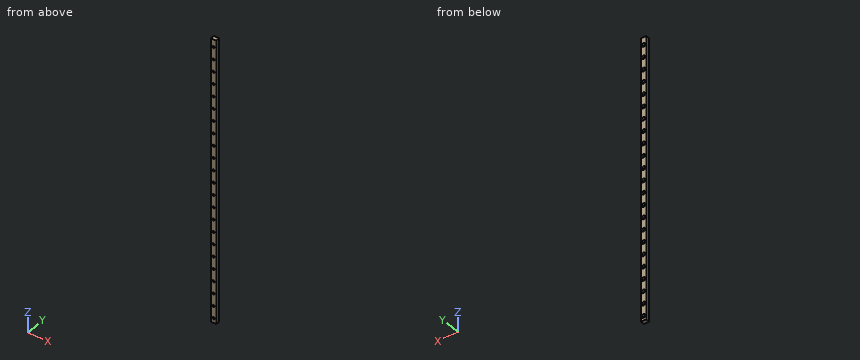
```python
from build123d import *

# Parameters (mm, degrees)
SKETCH_1_W          = 9
SKETCH_1_H          = 6.5
EXTRUDE_1_DEPTH     = 460
SKETCH_2_R          = 1.750000006
CUT_EXTRUDE_1_DEPTH = 371.819449874
SKETCH_3_R          = 3.000000006
CUT_EXTRUDE_2_DEPTH = 3.5


with BuildPart() as part:
    # 草图1 → 凸台-拉伸1 (new body)
    with BuildSketch(Plane.XY.offset(-89.264832522)):
        Rectangle(SKETCH_1_W, SKETCH_1_H)
    extrude(amount=EXTRUDE_1_DEPTH)

    # 草图2 → 切除-拉伸1 (cut, through all)
    with BuildSketch(Plane(origin=(0, 3.25, 0), x_dir=(1, 0, 0), z_dir=(0, 1, 0))):
        with Locations(Location((0, 81.764832522, 0), (0, 0, 270))):
            Circle(SKETCH_2_R)
        with Locations(Location((0, 61.764832522, 0), (0, 0, 270))):
            Circle(SKETCH_2_R)
        with Locations(Location((0, 41.764832522, 0), (0, 0, 270))):
            Circle(SKETCH_2_R)
        with Locations(Location((0, 21.764832522, 0), (0, 0, 270))):
            Circle(SKETCH_2_R)
        with Locations(Location((0, 1.764832522, 0), (0, 0, 270))):
            Circle(SKETCH_2_R)
        with Locations(Location((0, -18.235167478, 0), (0, 0, 270))):
            Circle(SKETCH_2_R)
        with Locations(Location((0, -38.235167478, 0), (0, 0, 270))):
            Circle(SKETCH_2_R)
        with Locations(Location((0, -58.235167478, 0), (0, 0, 270))):
            Circle(SKETCH_2_R)
        with Locations(Location((0, -78.235167478, 0), (0, 0, 270))):
            Circle(SKETCH_2_R)
        with Locations(Location((0, -98.235167478, 0), (0, 0, 270))):
            Circle(SKETCH_2_R)
        with Locations(Location((0, -118.235167478, 0), (0, 0, 270))):
            Circle(SKETCH_2_R)
        with Locations(Location((0, -138.235167478, 0), (0, 0, 270))):
            Circle(SKETCH_2_R)
        with Locations(Location((0, -158.235167478, 0), (0, 0, 270))):
            Circle(SKETCH_2_R)
        with Locations(Location((0, -178.235167478, 0), (0, 0, 270))):
            Circle(SKETCH_2_R)
        with Locations(Location((0, -198.235167478, 0), (0, 0, 270))):
            Circle(SKETCH_2_R)
        with Locations(Location((0, -218.235167478, 0), (0, 0, 270))):
            Circle(SKETCH_2_R)
        with Locations(Location((0, -238.235167478, 0), (0, 0, 270))):
            Circle(SKETCH_2_R)
        with Locations(Location((0, -258.235167478, 0), (0, 0, 270))):
            Circle(SKETCH_2_R)
        with Locations(Location((0, -278.235167478, 0), (0, 0, 270))):
            Circle(SKETCH_2_R)
        with Locations(Location((0, -298.235167478, 0), (0, 0, 270))):
            Circle(SKETCH_2_R)
        with Locations(Location((0, -318.235167478, 0), (0, 0, 270))):
            Circle(SKETCH_2_R)
        with Locations(Location((0, -338.235167478, 0), (0, 0, 270))):
            Circle(SKETCH_2_R)
        with Locations(Location((0, -358.235167478, 0), (0, 0, 270))):
            Circle(SKETCH_2_R)
        with Locations((0, -378.235167478)):
            Circle(SKETCH_2_R)
        with Locations((0, -398.235167478)):
            Circle(SKETCH_2_R)
        with Locations((0, -418.235167478)):
            Circle(SKETCH_2_R)
        with Locations((0, -438.235167478)):
            Circle(SKETCH_2_R)
        with Locations((0, -458.235167478)):
            Circle(SKETCH_2_R)
        with Locations((0, -478.235167478)):
            Circle(SKETCH_2_R)
        with Locations((0, -498.235167478)):
            Circle(SKETCH_2_R)
        with Locations((0, -518.235167478)):
            Circle(SKETCH_2_R)
        with Locations((0, -538.235167478)):
            Circle(SKETCH_2_R)
        with Locations((0, -558.235167478)):
            Circle(SKETCH_2_R)
        with Locations((0, -578.235167478)):
            Circle(SKETCH_2_R)
        with Locations((0, -598.235167478)):
            Circle(SKETCH_2_R)
        with Locations((0, -618.235167478)):
            Circle(SKETCH_2_R)
        with Locations((0, -638.235167478)):
            Circle(SKETCH_2_R)
        with Locations((0, -658.235167478)):
            Circle(SKETCH_2_R)
        with Locations((0, -678.235167478)):
            Circle(SKETCH_2_R)
        with Locations((0, -698.235167478)):
            Circle(SKETCH_2_R)
        with Locations((0, -718.235167478)):
            Circle(SKETCH_2_R)
        with Locations((0, -738.235167478)):
            Circle(SKETCH_2_R)
        with Locations((0, -758.235167478)):
            Circle(SKETCH_2_R)
        with Locations((0, -778.235167478)):
            Circle(SKETCH_2_R)
        with Locations((0, -798.235167478)):
            Circle(SKETCH_2_R)
        with Locations((0, -818.235167478)):
            Circle(SKETCH_2_R)
        with Locations((0, -838.235167478)):
            Circle(SKETCH_2_R)
        with Locations((0, -858.235167478)):
            Circle(SKETCH_2_R)
        with Locations((0, -878.235167478)):
            Circle(SKETCH_2_R)
        with Locations((0, -898.235167478)):
            Circle(SKETCH_2_R)
        with Locations((0, -918.235167478)):
            Circle(SKETCH_2_R)
        with Locations((0, -938.235167478)):
            Circle(SKETCH_2_R)
        with Locations((0, -958.235167478)):
            Circle(SKETCH_2_R)
        with Locations((0, -978.235167478)):
            Circle(SKETCH_2_R)
        with Locations((0, -998.235167478)):
            Circle(SKETCH_2_R)
        with Locations((0, -1018.235167478)):
            Circle(SKETCH_2_R)
        with Locations((0, -1038.235167478)):
            Circle(SKETCH_2_R)
        with Locations((0, -1058.235167478)):
            Circle(SKETCH_2_R)
        with Locations((0, -1078.235167478)):
            Circle(SKETCH_2_R)
        with Locations((0, -1098.235167478)):
            Circle(SKETCH_2_R)
    extrude(amount=-CUT_EXTRUDE_1_DEPTH, mode=Mode.SUBTRACT)

    # 草图3 → 切除-拉伸2 (cut)
    with BuildSketch(Plane(origin=(0, 3.25, 0), x_dir=(1, 0, 0), z_dir=(0, 1, 0))):
        with Locations(Location((0, 81.764832522, 0), (0, 0, 270))):
            Circle(SKETCH_3_R)
        with Locations(Location((0, 61.764832522, 0), (0, 0, 270))):
            Circle(SKETCH_3_R)
        with Locations(Location((0, 41.764832522, 0), (0, 0, 270))):
            Circle(SKETCH_3_R)
        with Locations(Location((0, 21.764832522, 0), (0, 0, 270))):
            Circle(SKETCH_3_R)
        with Locations(Location((0, 1.764832522, 0), (0, 0, 270))):
            Circle(SKETCH_3_R)
        with Locations(Location((0, -18.235167478, 0), (0, 0, 270))):
            Circle(SKETCH_3_R)
        with Locations(Location((0, -38.235167478, 0), (0, 0, 270))):
            Circle(SKETCH_3_R)
        with Locations(Location((0, -58.235167478, 0), (0, 0, 270))):
            Circle(SKETCH_3_R)
        with Locations(Location((0, -78.235167478, 0), (0, 0, 270))):
            Circle(SKETCH_3_R)
        with Locations(Location((0, -98.235167478, 0), (0, 0, 270))):
            Circle(SKETCH_3_R)
        with Locations(Location((0, -118.235167478, 0), (0, 0, 270))):
            Circle(SKETCH_3_R)
        with Locations(Location((0, -138.235167478, 0), (0, 0, 270))):
            Circle(SKETCH_3_R)
        with Locations(Location((0, -158.235167478, 0), (0, 0, 270))):
            Circle(SKETCH_3_R)
        with Locations(Location((0, -178.235167478, 0), (0, 0, 270))):
            Circle(SKETCH_3_R)
        with Locations(Location((0, -198.235167478, 0), (0, 0, 270))):
            Circle(SKETCH_3_R)
        with Locations(Location((0, -218.235167478, 0), (0, 0, 270))):
            Circle(SKETCH_3_R)
        with Locations(Location((0, -238.235167478, 0), (0, 0, 270))):
            Circle(SKETCH_3_R)
        with Locations(Location((0, -258.235167478, 0), (0, 0, 270))):
            Circle(SKETCH_3_R)
        with Locations(Location((0, -278.235167478, 0), (0, 0, 270))):
            Circle(SKETCH_3_R)
        with Locations(Location((0, -298.235167478, 0), (0, 0, 270))):
            Circle(SKETCH_3_R)
        with Locations(Location((0, -318.235167478, 0), (0, 0, 270))):
            Circle(SKETCH_3_R)
        with Locations(Location((0, -338.235167478, 0), (0, 0, 270))):
            Circle(SKETCH_3_R)
        with Locations(Location((0, -358.235167478, 0), (0, 0, 270))):
            Circle(SKETCH_3_R)
        with Locations((0, -378.235167478)):
            Circle(SKETCH_3_R)
        with Locations((0, -398.235167478)):
            Circle(SKETCH_3_R)
        with Locations((0, -418.235167478)):
            Circle(SKETCH_3_R)
        with Locations((0, -438.235167478)):
            Circle(SKETCH_3_R)
        with Locations((0, -458.235167478)):
            Circle(SKETCH_3_R)
        with Locations((0, -478.235167478)):
            Circle(SKETCH_3_R)
        with Locations((0, -498.235167478)):
            Circle(SKETCH_3_R)
        with Locations((0, -518.235167478)):
            Circle(SKETCH_3_R)
        with Locations((0, -538.235167478)):
            Circle(SKETCH_3_R)
        with Locations((0, -558.235167478)):
            Circle(SKETCH_3_R)
        with Locations((0, -578.235167478)):
            Circle(SKETCH_3_R)
        with Locations((0, -598.235167478)):
            Circle(SKETCH_3_R)
        with Locations((0, -618.235167478)):
            Circle(SKETCH_3_R)
        with Locations((0, -638.235167478)):
            Circle(SKETCH_3_R)
        with Locations((0, -658.235167478)):
            Circle(SKETCH_3_R)
        with Locations((0, -678.235167478)):
            Circle(SKETCH_3_R)
        with Locations((0, -698.235167478)):
            Circle(SKETCH_3_R)
        with Locations((0, -718.235167478)):
            Circle(SKETCH_3_R)
        with Locations((0, -738.235167478)):
            Circle(SKETCH_3_R)
        with Locations((0, -758.235167478)):
            Circle(SKETCH_3_R)
        with Locations((0, -778.235167478)):
            Circle(SKETCH_3_R)
        with Locations((0, -798.235167478)):
            Circle(SKETCH_3_R)
        with Locations((0, -818.235167478)):
            Circle(SKETCH_3_R)
        with Locations((0, -838.235167478)):
            Circle(SKETCH_3_R)
        with Locations((0, -858.235167478)):
            Circle(SKETCH_3_R)
        with Locations((0, -878.235167478)):
            Circle(SKETCH_3_R)
        with Locations((0, -898.235167478)):
            Circle(SKETCH_3_R)
        with Locations((0, -918.235167478)):
            Circle(SKETCH_3_R)
        with Locations((0, -938.235167478)):
            Circle(SKETCH_3_R)
        with Locations((0, -958.235167478)):
            Circle(SKETCH_3_R)
        with Locations((0, -978.235167478)):
            Circle(SKETCH_3_R)
        with Locations((0, -998.235167478)):
            Circle(SKETCH_3_R)
        with Locations((0, -1018.235167478)):
            Circle(SKETCH_3_R)
        with Locations((0, -1038.235167478)):
            Circle(SKETCH_3_R)
        with Locations((0, -1058.235167478)):
            Circle(SKETCH_3_R)
        with Locations((0, -1078.235167478)):
            Circle(SKETCH_3_R)
        with Locations((0, -1098.235167478)):
            Circle(SKETCH_3_R)
    extrude(amount=-CUT_EXTRUDE_2_DEPTH, mode=Mode.SUBTRACT)


solid = part.part
```
Build history of the part. All positions in model axes, mm. Give positions to 0.01 mm unless a question says otherwise; leave off trailing zeros.
1) Drop a flat-ended pin along its axis: P1, Ø4, axis at x = 0, z = -81.76, coming from the +Y side. Give the stop position or say it passes through.
Values follow:
P1: stops at y = -0.25
2) Band-saw the part on A-A on x = 0. State how many separate pieces and enclosed holes the cut face has, then the cut area to 3 significant figures.
Values follow:
separate pieces: 24
enclosed holes: 0
area: 2,270 mm2
3) Probe line 1 along X through (y, z) = (0.5, 98.5); line 2 along X through (y, z) = (0.5, -0.5). List the from-to ranges inside material, lowest first.
Values follow:
line 1: x = -4.5 to -2.99, 2.99 to 4.5
line 2: x = -4.5 to -2.72, 2.72 to 4.5
